Check sheet for the modelled part. Datum: model origin and axes. Units: mm. A direction names the side the tool comes from. Round coordinates to 2 decimals unless told otherwise and drop trailing zeros. Loops run counter-clockwise (first coordinate to the right, second up) from the corner with the lowest first, then second, coordinate; pieces in that order, holes last. Notation, with made-up numbers: M 59.5,-5.5 L 81.5,-5.5 A7 ccw 81.5,-1.5 Z; hole C -39,-8.75 d8. An arc over 180 degrees is marked long. One line per question, with ' | ' between items. Start each with the question number.
(1) Section check A-A (x = -25). Record the boundary of the cut face in (y, z).
(2) Section check C-C (x = -6.5). Record the boundary of the cut face in (y, z), and give its area (3 significant figures).
(3) Thickness scan on probe 1 along Y at (x, z) = (-23.25, 7.5); probe 2 along Z at (x, y) = (-25, -2.05); probe 3 along Z at (x, y) = (-24.5, -8.75). Record the ranges inside material, lowest first. Write a range as [from, to].
(4) Section check B-B (z = 10). Record the boundary of the cut face in (x, y).
(5) Tool access check on faces 4 (the face through (-15, -12, 3)), 5 (the face through (-15, -23, 3)), 6 (the face through (-14.79, -20.15, 2.66)). Record the directions out of +Z, -Z, +X, -X, +Y, -Y that give a thin tool (end or side, any length) a straight path to the whole face; none if there is none.
(6) Draft check along Y on faces 1 (the face through (-15, -1, 15)), 2 (the face through (-15, 0, 7)), 3 (the face through (-15, -20, 5)). Enter one of: +Y half, -Y half, draft (parallel to the pull), parting line (faces both ways), or undercut.
(7) Section check D-D (y = -13.5). Record the boundary of the cut face in (x, z).
(8) Go/stop test with flat-tipped pins: P1, Ø3, axis at x = -5, z = 11, coming from the -Y side; P2, Ø1.5, axis at x = -18.5, y = -20, coming from the +Z side. Record where each tip stops, or that it passes through.
```python
from build123d import *

# Parameters (mm, degrees)
F1_DEPTH = 30
F3_D     = 1.5
F5_DEPTH = 30


with BuildPart() as f1:
    # F0 (on Right) → F1 (new body)
    with BuildSketch(Plane.YZ):
        Polygon((-20, 0), (0, 0), (0, 15), (-3, 15), (-3, 5), (-5, 3), (-20, 3), align=None)
        with BuildLine():
            ThreePointArc((-20, 6), (-23, 3), (-20, 0))
            Line((-20, 0), (-20, 3))
            Line((-20, 3), (-20, 6))
        make_face()
    extrude(amount=-F1_DEPTH)

    # F3 (through all)
    with Locations(Plane.XZ.offset(3)):
        with Locations((-25, 10), (-5, 10)):
            Hole(F3_D / 2)

    # F4 (on face) → F5 (cut)
    with BuildSketch(Plane.YZ):
        Polygon((-19.5, 3), (-20, 3), (-20, 1.5), align=None)
        Polygon((-20, 1.5), (-20, 3), (-20, 3.4), (-20.3, 1.9), align=None)
    extrude(amount=-F5_DEPTH, mode=Mode.SUBTRACT)


solid = f1.part
```
The answers:
1) outline: M -20.3,1.9 L -20,3.4 L -20,6 A3 ccw -20,0 L 0,0 L 0,9.25 L -3,9.25 L -3,5 L -5,3 L -19.5,3 L -20,1.5 Z; M -3,10.75 L 0,10.75 L 0,15 L -3,15 Z
2) outline: M -20.3,1.9 L -20,3.4 L -20,6 A3 ccw -20,0 L 0,0 L 0,15 L -3,15 L -3,5 L -5,3 L -19.5,3 L -20,1.5 Z | area: 111 mm²
3) probe 1: [-3, 0] | probe 2: [0, 9.25], [10.75, 15] | probe 3: [0, 3]
4) outline: M -30,-3 L -25.75,-3 L -25.75,0 L -30,0 Z; M -24.25,-3 L -5.75,-3 L -5.75,0 L -24.25,0 Z; M -4.25,-3 L 0,-3 L 0,0 L -4.25,0 Z
5) face 4: +Z, +X, -X | face 5: +X, -X, -Y | face 6: +X, -X
6) face 1: draft | face 2: +Y half | face 3: undercut
7) outline: M -30,0 L 0,0 L 0,3 L -30,3 Z
8) P1: y = -3 | P2: z = 6
